Job drawing, mm, ordinate dimensions from the low corner. One solid piece. Round coordinates to 2 decimals unless told otherwise and drop trailing zeros. Loops run counter-clockwise (first coordinate to the right, second up) from the corner with the lowest first, then second, coordinate; pieces in that order, holes last.
1) Probe line 1 (Y direction, x = 268, z = 0.9). List the from-to ranges inside material, lowest first.
2) Band-saw the part on A-A, the plane y = 78. Write the cut outline in (x, z), then the cut area to 3 significant figures.
3) Drop flat-ended pins along their axis: P1, Ø2, axis at x = 32, z = 1.5, coming from the +Y side; P2, Ø1.2, axis at y = 260, z = 1, coming from the +X side. Give the stop position or say it passes through.
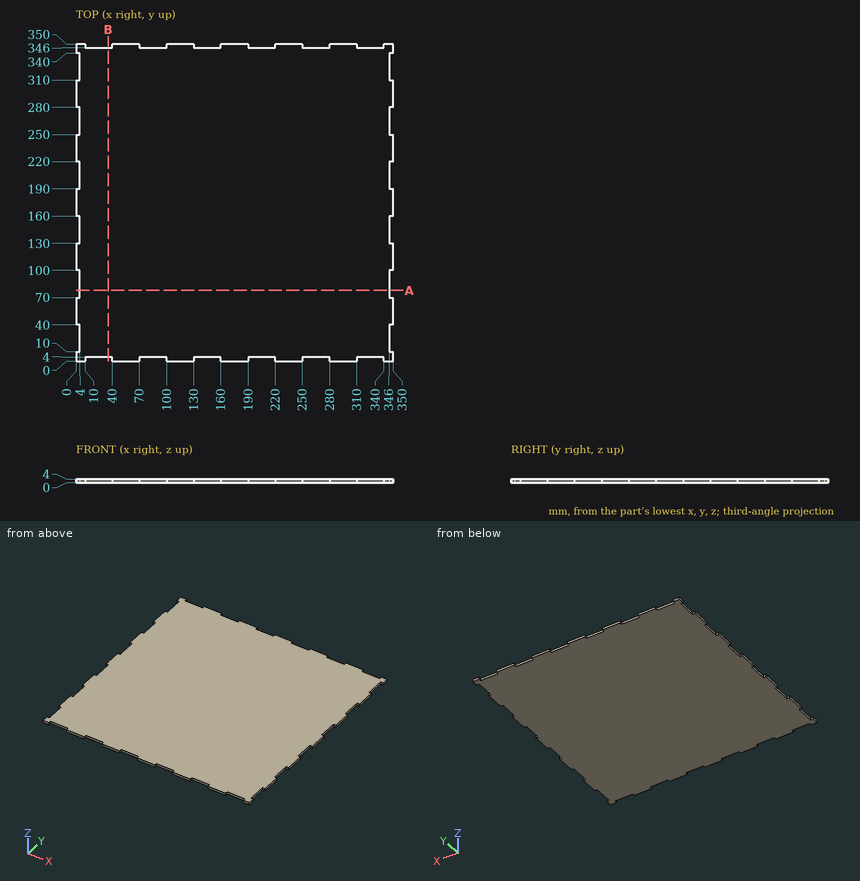
Reported:
1. line 1: y = 4 to 346
2. outline: (4, 0) - (346, 0) - (346, 4) - (4, 4) - close
2. area: 1,370 mm2
3. P1: stops at y = 346
3. P2: stops at x = 346
